```python
from build123d import *

# Parameters (mm, degrees)
BASE_FLANGE_DEPTH         = 31.75
MITER_FLANGE2_DEPTH       = 88.9
MITER_FLANGE2_2_DEPTH     = 3.175
MITER_START               = 3.175
MITER_FLANGE2_3_DEPTH     = 85.725
MITER_START_2             = -19.05
MITER_FLANGE2_4_OUTLINE_W = 19.05
MITER_FLANGE2_4_OUTLINE_H = 1.5875
MITER_FLANGE2_4_DEPTH     = 17.4625
MITER_FLANGE2_5_DEPTH     = 19.05
MITER_FLANGE2_6_DEPTH     = 19.05
CUT_EXTRUDE5_DEPTH        = 1.5875
CUT_EXTRUDE2_REACH        = 105.029
SKETCH5_R                 = 2.54
CUT_EXTRUDE4_REACH        = 107.049
SKETCH7_R                 = 2.54


with BuildPart() as part:
    # Base-Flange: sheet metal written as solids
    # Sketch1 → Base-Flange (new body)
    with BuildSketch(Plane.XY):
        with BuildLine():
            Line((0, 0), (19.05, 0))
            ThreePointArc((19.05, 0), (21.29506403, 0.92993597), (22.225, 3.175))
            Line((22.225, 3.175), (22.225, 88.9))
            Line((22.225, 88.9), (20.6375, 88.9))
            Line((20.6375, 88.9), (20.6375, 3.175))
            ThreePointArc((20.6375, 3.175), (20.172532015, 2.052467985), (19.05, 1.5875))
            Line((19.05, 1.5875), (0, 1.5875))
            Line((0, 1.5875), (0, 0))
        make_face()
    extrude(amount=BASE_FLANGE_DEPTH)

    # Miter Flange2: read off the stored shape, not the designer's step
    # Miter Flange2 outline → Miter Flange2 (cut)
    with BuildSketch(Plane(origin=(0, 0, 0), x_dir=(1, 0, 0), z_dir=(0, 1, 0))):
        with BuildLine():
            Line((22.225, 0), (19.05, 0))
            Line((19.05, 0), (19.05, -3.175))
            Line((19.05, -3.175), (20.6375, -3.175))
            ThreePointArc((20.6375, -3.175), (21.062869343, -1.5875), (22.225, -0.425369343))
            Line((22.225, -0.425369343), (22.225, 0))
        make_face()
    extrude(amount=MITER_FLANGE2_DEPTH, mode=Mode.SUBTRACT)

    # Miter Flange2 2 outline → Miter Flange2 2 (cut)
    with BuildSketch(Plane(origin=(0, 0, 0), x_dir=(1, 0, 0), z_dir=(0, 1, 0))):
        with BuildLine():
            Line((20.6375, -3.175), (22.225, -3.175))
            Line((22.225, -3.175), (22.225, -0.425369343))
            ThreePointArc((22.225, -0.425369343), (21.062869343, -1.5875), (20.6375, -3.175))
        make_face()
    extrude(amount=MITER_FLANGE2_2_DEPTH, mode=Mode.SUBTRACT)

    # Miter Flange2 3 outline → Miter Flange2 3 (add)
    with BuildSketch(Plane(origin=(0, 0, 0), x_dir=(1, 0, 0), z_dir=(0, 1, 0)).offset(MITER_START)):
        with BuildLine():
            Line((22.225, -0.425369343), (22.225, -3.175))
            ThreePointArc((22.225, -3.175), (22.689967985, -2.052467985), (23.8125, -1.5875))
            Line((23.8125, -1.5875), (41.275, -1.5875))
            Line((41.275, -1.5875), (41.275, 0))
            Line((41.275, 0), (23.8125, 0))
            ThreePointArc((23.8125, 0), (22.990749532, -0.108185502), (22.225, -0.425369343))
        make_face()
    extrude(amount=MITER_FLANGE2_3_DEPTH)

    # Miter Flange2 5 outline → Miter Flange2 5 (cut)
    with BuildSketch(Plane.YZ):
        with BuildLine():
            ThreePointArc((1.5875, 3.175), (1.162130657, 1.5875), (0, 0.425369343))
            Line((0, 0.425369343), (0, 0))
            Line((0, 0), (1.5875, 0))
            Line((1.5875, 0), (1.5875, 3.175))
        make_face()
    extrude(amount=MITER_FLANGE2_5_DEPTH, mode=Mode.SUBTRACT)



with BuildPart() as body_2:
    # Miter Flange2 4 outline → Miter Flange2 4 (new body)
    with BuildSketch(Plane(origin=(0, 0, 0), x_dir=(1, 0, 0), z_dir=(0, 1, 0)).offset(MITER_START_2)):
        with Locations((9.525, -0.79375)):
            Rectangle(MITER_FLANGE2_4_OUTLINE_W, MITER_FLANGE2_4_OUTLINE_H)
    extrude(amount=MITER_FLANGE2_4_DEPTH)


with BuildPart() as part_1:
    add(part.part)

    add(body_2.part)  # Miter Flange2 6 merges body 2
    # Miter Flange2 6 outline → Miter Flange2 6 (add)
    with BuildSketch(Plane.YZ):
        with BuildLine():
            Line((0, 0.425369343), (0, 3.175))
            ThreePointArc((0, 3.175), (-0.464967985, 2.052467985), (-1.5875, 1.5875))
            Line((-1.5875, 1.5875), (-1.5875, 0))
            ThreePointArc((-1.5875, 0), (-0.765749532, 0.108185502), (0, 0.425369343))
        make_face()
    extrude(amount=MITER_FLANGE2_6_DEPTH)

    # Sketch8 → Cut-Extrude5 (cut)
    with BuildSketch(Plane.XY.offset(1.5875)):
        with BuildLine():
            Line((32.385, 76.2), (32.385, 28.575))
            ThreePointArc((32.385, 28.575), (34.925, 26.035), (37.465, 28.575))
            Line((37.465, 28.575), (37.465, 76.2))
            ThreePointArc((37.465, 76.2), (34.925, 78.74), (32.385, 76.2))
        make_face()
    extrude(amount=-CUT_EXTRUDE5_DEPTH, mode=Mode.SUBTRACT)

    # Sketch5 → Cut-Extrude2 (cut, up to next)
    with BuildSketch(Plane(origin=(0, 0, 0), x_dir=(-1, 0, 0), z_dir=(0, 0, -1)), mode=Mode.PRIVATE) as cut_extrude2_sk1:
        with Locations((-12.7, -12.7)):
            Circle(SKETCH5_R)
    cut_extrude2_tool1 = extrude(cut_extrude2_sk1.sketch, amount=-CUT_EXTRUDE2_REACH, mode=Mode.PRIVATE) & part_1.part
    add(cut_extrude2_tool1.solids().sort_by_distance((12.7, -12.7, 0))[0], mode=Mode.SUBTRACT)

    # Sketch7 → Cut-Extrude4 (cut, up to next)
    with BuildSketch(Plane(origin=(22.225, -0.213353633, 50.991788494), x_dir=(0, 0, -1), z_dir=(1, 0, 0)), mode=Mode.PRIVATE) as cut_extrude4_sk1:
        with Locations(Location((25.591788494, 76.413353633, 0), (0, 0, 90))):
            Circle(SKETCH7_R)
    cut_extrude4_tool1 = extrude(cut_extrude4_sk1.sketch, amount=-CUT_EXTRUDE4_REACH, mode=Mode.PRIVATE) & part_1.part
    # Sketch7 → Cut-Extrude4 (cut, up to next)
    with BuildSketch(Plane(origin=(22.225, -0.213353633, 50.991788494), x_dir=(0, 0, -1), z_dir=(1, 0, 0)), mode=Mode.PRIVATE) as cut_extrude4_sk2:
        with Locations(Location((25.591788494, 46.250853633, 0), (0, 0, 90))):
            Circle(SKETCH7_R)
    cut_extrude4_tool2 = extrude(cut_extrude4_sk2.sketch, amount=-CUT_EXTRUDE4_REACH, mode=Mode.PRIVATE) & part_1.part
    # Sketch7 → Cut-Extrude4 (cut, up to next)
    with BuildSketch(Plane(origin=(22.225, -0.213353633, 50.991788494), x_dir=(0, 0, -1), z_dir=(1, 0, 0)), mode=Mode.PRIVATE) as cut_extrude4_sk3:
        with Locations(Location((25.591788494, 16.088353633, 0), (0, 0, 90))):
            Circle(SKETCH7_R)
    cut_extrude4_tool3 = extrude(cut_extrude4_sk3.sketch, amount=-CUT_EXTRUDE4_REACH, mode=Mode.PRIVATE) & part_1.part
    add(cut_extrude4_tool1.solids().sort_by_distance((22.225, 76.2, 25.4))[0], mode=Mode.SUBTRACT)
    add(cut_extrude4_tool2.solids().sort_by_distance((22.225, 46.0375, 25.4))[0], mode=Mode.SUBTRACT)
    add(cut_extrude4_tool3.solids().sort_by_distance((22.225, 15.875, 25.4))[0], mode=Mode.SUBTRACT)

    # SHM-Mirror1: part across plane


with BuildPart() as part_2:
    add(part_1.part)
    add(part_1.part.mirror(Plane(origin=(0, 0, 31.75), x_dir=(0, 0, 1), z_dir=(-1, 0, 0))))


solid = part_2.part
```
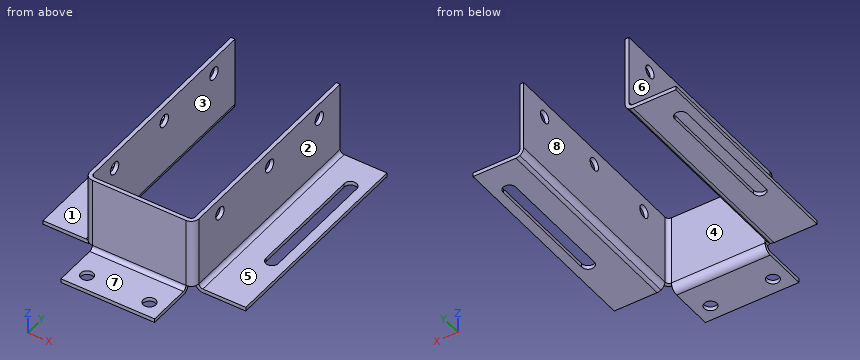
Read the model definition and answer for the solid it produces. Units are mm, in the model's axes. Face numbers are marked on the shaded views. A direction names the side the tool comes from. Coordinates: 2 decimals unless noted, no trailing zeros. Loops run counter-clockwise (first coordinate to the right, second up) from the corner with the lowest first, then second, coordinate; pieces in that order, holes last. Notation, with made-up numbers: (-6.75, 3) -> (24.25, 3) arc R24 ccw to (24.25, 28) -> close; hole circle Ø9 at (83.5, 11). An arc over 180 degrees is marked (long way). Return JSON: item names as keys, results as strings.
Item 1: Find section C-C (y = -12.7). Determine the outline of the cut face in (x, z).
Answers:
{"outline": "(-19.05, 0) -> (-15.24, 0) -> (-15.24, 1.59) -> (-19.05, 1.59) -> close; (-10.16, 0) -> (10.16, 0) -> (10.16, 1.59) -> (-10.16, 1.59) -> close; (15.24, 0) -> (19.05, 0) -> (19.05, 1.59) -> (15.24, 1.59) -> close"}
Item 2: Find section A-A (y = 56.5). Count the separate pieces of the cut face and the enclosed holes in it, plus the area to 3 significant figures.
Answers:
{"separate pieces": "4", "enclosed holes": "0", "area": "142 mm2"}
Item 3: Find the intervals of material crossed by probe 1 along X at (y, z) = (78.5, 20) (1 decimal); probe 2 along X at (y, z) = (-12, 1); probe 3 along Y at (x, z) = (21, 25), in increasing order.
Answers:
{"probe 1": "x = -22.2 to -20.6, 20.6 to 22.2", "probe 2": "x = -19.05 to -15.14, -10.26 to 10.26, 15.14 to 19.05", "probe 3": "y = 0.67 to 13.37, 18.38 to 43.53, 48.55 to 73.69, 78.71 to 88.9"}
Item 4: For a pull along X with two mould halves and no side action, classify the marked faces 1, 2, 3 and 4 as +X half, -X half, draft (parallel to the pull), parting line (faces both ways), or undercut.
Answers:
{"face 1": "draft", "face 2": "+X half", "face 3": "undercut", "face 4": "undercut"}
Item 5: Flat-ended cylindrical pins translate along their axes: P1, Ø1.6, axis at y = -8, z = 1, coming from the -X side; P2, Ø1.5, axis at x = 17.5, z = 19.5, coming from the +Y side; P3, Ø3.5, axis at x = 21, y = 1, coming from the -Z side (3 decimals). Find the tip coordinate at first contact, or state that the pin passes through.
Answers:
{"P1": "stops at x = -19.05", "P2": "stops at y = 1.59", "P3": "stops at z = 3.175"}
Item 6: For the marked faces 5, 6, 7 and 8, determine the directions among +Z, -Z, +X, -X, +Y, -Y from which every point of the face is accessible in a straight line to the end or side of a thin tool.
Answers:
{"face 5": "+Z, +X, +Y, -Y", "face 6": "+Z, -X, +Y, -Y", "face 7": "+Z, +X, -X, -Y", "face 8": "+Z, -Z, +Y"}
